Part model, mm, in its own coordinate system. A direction names the side the tool comes from. Round coordinates to 2 decimals unless told otherwise and drop trailing zeros. Loops run counter-clockwise (first coordinate to the right, second up) from the corner with the lowest first, then second, coordinate; pieces in that order, holes last. Notation, with made-up numbers: (63, 43) -> (95, 43) arc R13 ccw to (95, 55) -> close; hole circle Ø4 at (54.25, -14.5). An arc over 180 degrees is marked (long way). Use a Markdown table: item, result. Add a question column.
Item 1: Cut at A-A, the plane x = 5.08. List the corners of the cut face in (y, z).
Item 2: Flat gauge pins, fed straight in: pin 1 (0.8 mm diameter, centred on y = 7, z = -1.5, fed in from +X); pin 2 (3 mm diameter, centred on x = 23.5, y = 6, fed in from +Z). Where does each tip first touch, or does it go through?
Item 3: Cut at D-D, the plane y = 5.08. List the corners of the cut face in (x, z).
Item 4: Which spindle directions (+Z, -Z, +X, -X, +Y, -Y) get a long thin tool onto all of the face, cutting with end or side? Do faces 4 (the face through (8, 6.35, -3)), 5 (the face through (31.77, 1.29, -4.42)), 6 (the face through (24, 5, -2.54)), 7 (the face through (7.85, 8.23, -4.81)), 8 (the face through (19.05, 5, -8)). Say none if no direction does.
Item 5: Cut at C-C, the plane z = -4.5. List the corners of the cut face in (x, y) (3 decimals), plus the area to 3 significant figures.
Item 6: Two-plate mould, pull along X, no slides. Class faces 1 (the face through (25.246, 6.968, -4.418)), 2 (the face through (19.05, 5, -1)), 3 (the face through (22, 0, -5)): pulls with the +X half, pulls with the -X half, needs draft (parallel to the pull), parting line crosses it, or undercut.
Item 7: Probe line 1 (Z direction, x = 5.08, y = 7.3); line 2 (X direction, y = 6.5, z = -5); line 3 (X direction, y = 7.25, z = -5.5). List the from-to ranges inside material, lowest first. Write a range as [from, to].
Item 8: Cut at B-B, the plane y = 3.5. List the corners of the cut face in (x, z), plus the area to 3 significant figures.
```python
from build123d import *

# Parameters (mm, degrees)
SKETCH1_R            = 2.794
BASE_DEPTH           = 10.16
LATCH_HOLE_REACH     = 37.126
SKETCH2_R            = 2.794
SERVO_ARM_HOLE_REACH = 37.673
CHAMFER1_SIZE        = 2.54


with BuildPart() as part:
    # Sketch1 → base (new body)
    with BuildSketch(Plane(origin=(0, 0, 0), x_dir=(1, 0, 0), z_dir=(0, 1, 0))):
        Polygon((0, 0), (19.05, 0), (19.05, 2.54), (33.02, 2.54), (33.02, 6.35), (19.05, 6.35), (19.05, 8.89), (0, 8.89), align=None)
        with Locations(Location((5.08, 4.445, 0), (0, 0, 270))):
            Circle(SKETCH1_R, mode=Mode.SUBTRACT)
    extrude(amount=BASE_DEPTH)

    # Sketch2 → latch_hole (cut, up to next)
    with BuildSketch(Plane.XY.offset(-2.54), mode=Mode.PRIVATE) as latch_hole_sk1:
        with Locations((27.305, 5.08)):
            Circle(SKETCH2_R)
    latch_hole_tool1 = extrude(latch_hole_sk1.sketch, amount=-LATCH_HOLE_REACH, mode=Mode.PRIVATE) & part.part
    add(latch_hole_tool1.solids().sort_by_distance((27.305, 5.08, -2.54))[0], mode=Mode.SUBTRACT)

    # Sketch4 → servo_arm_hole (cut, up to next)
    with BuildSketch(Plane.XY, mode=Mode.PRIVATE) as servo_arm_hole_sk1:
        Polygon((0, 6.35), (12.7, 6.35), (16.51, 0), (0, 0), align=None)
    servo_arm_hole_tool1 = extrude(servo_arm_hole_sk1.sketch, amount=-SERVO_ARM_HOLE_REACH, mode=Mode.PRIVATE) & part.part
    add(servo_arm_hole_tool1.solids().sort_by_distance((7.343913, 3.036957, 0))[0], mode=Mode.SUBTRACT)

    # Chamfer1
    chamfer1_edges = [part.edges().sort_by_distance(p)[0] for p in [
        (0, 8.255, -8.89),
        (0, 8.255, 0),
        (33.02, 10.16, -4.445),
        (33.02, 0, -4.445),
    ]]
    chamfer(chamfer1_edges, length=CHAMFER1_SIZE)


solid = part.part
```
A:
| question | item | result |
|---|---|---|
| 1 | outline | (6.35, -8.89) -> (10.16, -8.89) -> (10.16, -7.24) -> (6.35, -7.24) -> close; (6.35, -1.65) -> (10.16, -1.65) -> (10.16, 0) -> (6.35, 0) -> close |
| 2 | pin 1 | stops at x = 19.05 |
| 2 | pin 2 | stops at z = -2.54 |
| 3 | outline | (13.46, -8.89) -> (19.05, -8.89) -> (19.05, -6.35) -> (24.51, -6.35) -> (24.51, -2.54) -> (19.05, -2.54) -> (19.05, 0) -> (13.46, 0) -> close; (30.1, -6.35) -> (33.02, -6.35) -> (33.02, -2.54) -> (30.1, -2.54) -> close |
| 4 | face 4 | +Z, -Z, -X, -Y |
| 4 | face 5 | +Z, -Z, +X, -Y |
| 4 | face 6 | +Z, +X, +Y, -Y |
| 4 | face 7 | +Y, -Y |
| 4 | face 8 | -Z, +X, +Y, -Y |
| 5 | outline | (0, 6.35) -> (2.287, 6.35) -> (2.287, 10.16) -> (0, 10.16) -> close; (7.873, 6.35) -> (12.7, 6.35) -> (16.51, 0) -> (30.48, 0) -> (33.02, 2.54) -> (33.02, 7.62) -> (30.48, 10.16) -> (7.873, 10.16) -> close; hole circle Ø5.588 at (27.305, 5.08) |
| 5 | area | 190 mm^2 |
| 6 | face 1 | undercut |
| 6 | face 2 | pulls with the +X half |
| 6 | face 3 | needs draft |
| 7 | line 1 | z = [-8.89, -7.24], [-1.65, 0] |
| 7 | line 2 | x = [0, 2.34], [7.82, 24.9], [29.71, 33.02] |
| 7 | line 3 | x = [0, 2.49], [7.67, 25.55], [29.06, 33.02] |
| 8 | outline | (14.41, -8.89) -> (19.05, -8.89) -> (19.05, -6.35) -> (25, -6.35) -> (25, -2.54) -> (19.05, -2.54) -> (19.05, 0) -> (14.41, 0) -> close; (29.61, -6.35) -> (33.02, -6.35) -> (33.02, -2.54) -> (29.61, -2.54) -> close |
| 8 | area | 76.9 mm^2 |
